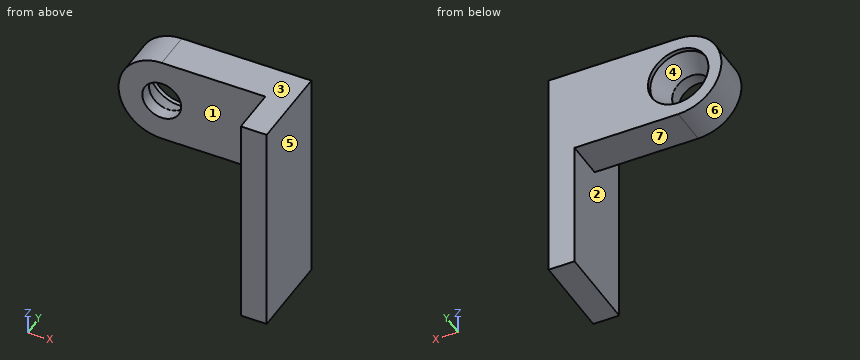
```python
from build123d import *

# Parameters (mm, degrees)
SKETCH1_R           = 2.25
BOSS_EXTRUDE1_DEPTH = 4.5
SKETCH2_W           = 25
SKETCH2_H           = 10
BOSS_EXTRUDE2_DEPTH = 3
SKETCH3_R           = 3.5
CUT_EXTRUDE1_DEPTH  = 3
CHAMFER1_SIZE2      = 1.25
CHAMFER1_SIZE       = 2.5


with BuildPart() as part:
    # Sketch1 → Boss-Extrude1 (new body)
    with BuildSketch(Plane(origin=(0, 0, 0), x_dir=(1, 0, 0), z_dir=(0, 1, 0))):
        with BuildLine():
            Line((0, 5), (15, 5))
            Line((15, 5), (15, -5))
            Line((15, -5), (0, -5))
            ThreePointArc((0, -5), (-5, 0), (0, 5))
        make_face()
        with Locations(Location((0, 0, 0), (0, 0, 270))):
            Circle(SKETCH1_R, mode=Mode.SUBTRACT)
    extrude(amount=BOSS_EXTRUDE1_DEPTH)

    # Sketch2 → Boss-Extrude2 (add)
    with BuildSketch(Plane(origin=(15, 0, 0), x_dir=(0, 0, -1), z_dir=(1, 0, 0))):
        with Locations((7.5, -0.5)):
            Rectangle(SKETCH2_W, SKETCH2_H)
    extrude(amount=-BOSS_EXTRUDE2_DEPTH)

    # Sketch3 → Cut-Extrude1 (cut)
    with BuildSketch(Plane(origin=(0, 4.5, 0), x_dir=(1, 0, 0), z_dir=(0, 1, 0))):
        with Locations(Location((0, 0, 0), (0, 0, 270))):
            Circle(SKETCH3_R)
    extrude(amount=-CUT_EXTRUDE1_DEPTH, mode=Mode.SUBTRACT)

    # Chamfer1
    chamfer1_edges = [part.edges().sort_by_distance(p)[0] for p in [
        (0, 1.5, -3.5),
    ]]
    chamfer1_side = [part.faces().sort_by_distance(p)[0] for p in [
        (0, 1.525, -3.5),
    ]]
    chamfer(chamfer1_edges, length=CHAMFER1_SIZE - 0.0001, length2=CHAMFER1_SIZE2 - 0.0001, reference=chamfer1_side[0])  # a hair under: the kernel refuses the full size


solid = part.part
```
CAD build for the part. Positions are in the model's coordinates, mm. Face numbers are marked on the shaded views. A direction names the side the tool comes from. Round coordinates to 2 decimals unless told otherwise and drop trailing zeros. Write each loop counter-clockwise with the first axis right and the second up, starting at its lowest first coordinate (ties: lowest second). Pieces come first, ordered by that corner, then holes. Notation, with made-up numbers: (73, -6.75) - (95, -6.75) arc R32 ccw to (95, 26.25) - close; hole circle Ø8 at (20.25, 11.5). An arc over 180 degrees is marked (long way). Write item = value, one per line. Start each with the question number.
Q1. Which spindle directions (+Z, -Z, +X, -X, +Y, -Y) get a long thin tool onto all of the face, cutting with end or side? Do the marked faces 1, 2 and 3. Say none if no direction does.
Q2. Band-saw the part on C-C (z = -14.5). Give the cut face in (x, y).
Q3. Band-saw the part on D-D (x = 8.75). Give the cut face in (y, z).
Q4. Probe L1, parallel to Z at x = 0, y = 0.4; L2, parallel to X at y = 4.1, z = 0; L3, parallel to X at y = 1, z = 0. List the from-to ranges inside material, lowest first. Write a range as from..to.
Q5. Band-saw the part on B-B (y = 0.5). Give the cut face in (x, z).
Q6. Mould opens along Z. For the marked faces 4, 5, 6 and 7 say: pulls with the +Z half, pulls with the -Z half, needs draft (parallel to the pull), parting line crosses it, or undercut.
Q7. Drop flat-ended pins along their axis: pin 1 (5 mm diameter, centred on y = 0.5, z = -3.5, fed in from -X); pin 2 (2.5 mm diameter, centred on x = 1, z = 1, fed in from +Y); pin 3 (6.5 mm diameter, centred on x = 0, z = 0, fed in from +Y); pin 4 (4 mm diameter, centred on x = 9, z = -10, fed in from -Y). Give the stop position or say it passes through.
Answers below:
q1.face_1 = +Z, -Z, -X, -Y
q1.face_2 = -Z, -X, -Y
q1.face_3 = +Z, +X, -X, +Y, -Y
q2.outline = (12, -5.5) - (15, -5.5) - (15, 4.5) - (12, 4.5) - close
q3.outline = (0, -5) - (4.5, -5) - (4.5, 5) - (0, 5) - close
q4.L1 = -5..-2.25, 2.25..5
q4.L2 = -5..-3.5, 3.5..15
q4.L3 = -5..-2.25, 2.25..15
q5.outline = (0, -5) - (12, -5) - (12, -20) - (15, -20) - (15, 5) - (0, 5) arc R5 ccw to start; hole circle Ø4.5 at (0, 0)
q6.face_4 = undercut
q6.face_5 = needs draft
q6.face_6 = parting line crosses it
q6.face_7 = pulls with the -Z half
q7.pin_1 = -4.9
q7.pin_2 = 2.33
q7.pin_3 = 3.5
q7.pin_4 = through
